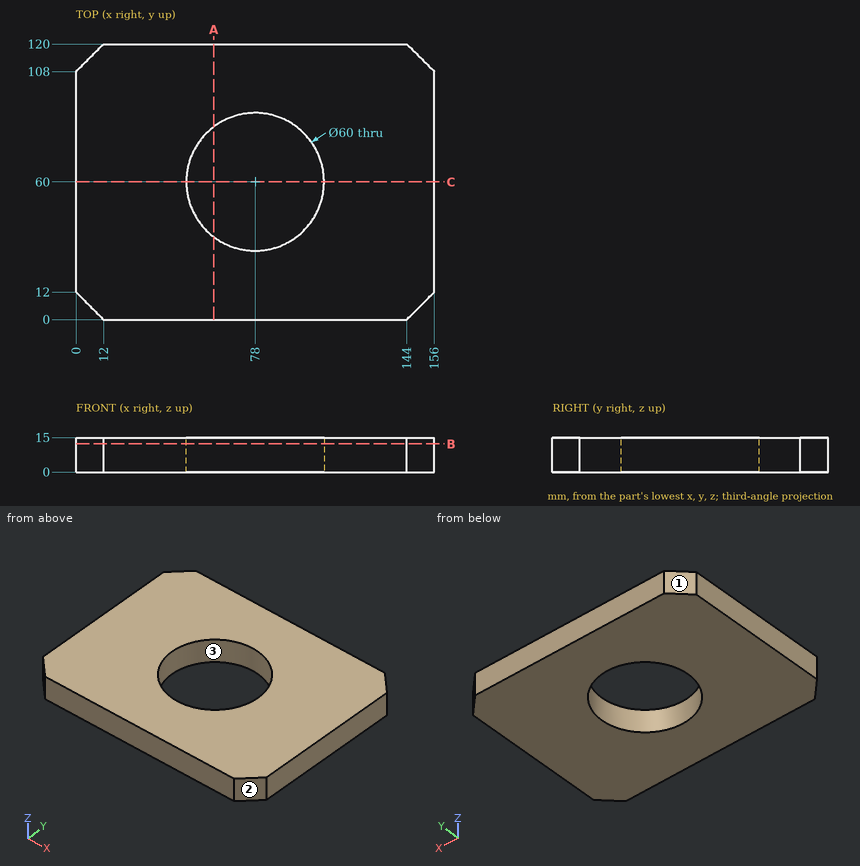
Part print with two shaded views. Sizes in mm from the minimum x, y, z corner. Coordinates: 2 decimals unless noted, no trailing zeros. Order: outer loops, then holes, each group sorted by start corner. A loop starts at its lowest first (then second) coordinate and runs counter-clockwise, first axis right, second up.
(1) Saw through at C-C, the plane y = 60. Write the cut outline in (x, z), and give its area (3 significant figures).
Solution:
outline: (0, 0) - (48, 0) - (48, 15) - (0, 15) - close; (108, 0) - (156, 0) - (156, 15) - (108, 15) - close
area: 1,440 mm2
(2) Drill centre lines: L1, parallel to Y at x = 78, z = 5.25; L2, parallel to X at y = 39, z = 2.25; L3, parallel to Y at x = 105, z = 0.75. Where is each one in solid material? Low to high.
Solution:
L1: y = 0 to 30, 90 to 120
L2: x = 0 to 56.58, 99.42 to 156
L3: y = 0 to 46.92, 73.08 to 120
(3) Saw through at A-A, the plane x = 60. Write the cut outline in (y, z), and give its area (3 significant figures).
Solution:
outline: (0, 0) - (36, 0) - (36, 15) - (0, 15) - close; (84, 0) - (120, 0) - (120, 15) - (84, 15) - close
area: 1,080 mm2
(4) Saw through at B-B, the plane z = 12.25. Write the cut outline in (x, y).
Solution:
outline: (0, 12) - (12, 0) - (144, 0) - (156, 12) - (156, 108) - (144, 120) - (12, 120) - (0, 108) - close; hole circle Ø60 at (78, 60)
(5) Mould opens along Y. For the marked faces 1, 2 and 3 say: released by +Y, released by -Y, zero draft, split by the parting line, or undercut.
Solution:
face 1: released by +Y
face 2: released by -Y
face 3: undercut
